Autodesk Inventor part; units mm, degrees
ref_plane "YZ Plane" through (0, 0, 0) normal (1, 0, 0) x (0, 1, 0)
ref_plane "XZ Plane" through (0, 0, 0) normal (0, 1, 0) x (-1, 0, 0)
ref_plane "XY Plane" through (0, 0, 0) normal (0, 0, 1) x (1, 0, 0)
sketch "草图1" plane through (0, 0, 0) normal (0, 1, 0) x (-1, 0, 0)
  line L0 (0, 0) -> (-8, 0)
  line L1 (-8, 0) -> (-8, -5)
  line L2 (-8, -5) -> (0, -5)
  line L3 (0, -5) -> (0, 0)
  line L4 (0, -5) -> (-5, -5)
  line L5 (-5, -5) -> (-5, -7.5)
  line L6 (-5, -7.5) -> (0, -7.5)
  line L7 (0, -7.5) -> (0, -5)
  line L8 (0, -7.5) -> (-5.75, -7.5)
  line L9 (-5.75, -7.5) -> (-5.75, -45)
  line L10 (-5.75, -45) -> (0, -45)
  line L11 (0, -45) -> (0, -7.5)
  line L12 (0, -45) -> (-5.25, -45)
  line L13 (-5.25, -45) -> (-5.25, -46.1)
  line L14 (-5.25, -46.1) -> (0, -46.1)
  line L15 (0, -46.1) -> (0, -45)
  line L16 (0, -46.1) -> (-5.75, -46.1)
  line L17 (-5.75, -46.1) -> (-5.75, -50)
  line L18 (-5.75, -50) -> (0, -50)
  line L19 (0, -50) -> (0, -46.1)
  dimension "d0" = 8
  dimension "d1" = 5
  dimension "d2" = 5
  dimension "d3" = 2.5
  dimension "d4" = 5.75
  dimension "d5" = 37.5
  dimension "d6" = 5.25
  dimension "d7" = 1.1
  dimension "d8" = 5.75
  dimension "d9" = 3.9
revolve "旋转1" add sketch "草图1" angle 360 about axis through (0, 0, -45) along (0, 0, 1)
fillet "圆角1" radius 1 2 edges at (-8, 0, 0) (-5.75, 0, -50)
properties part number "6-鞘轴" material "不锈钢"
Source: CAD feature listing. Evaluate the final solid. Frame: model axes, mm. A direction names the side the tool comes from. Give positions to 0.01 mm unless a question says otherwise; leave off trailing zeros. Order: outer loops, then holes, each group sorted by start corner. A loop starts at its lowest first (then second) coordinate and runs counter-clockwise, first axis right, second up. Notation, with made-up numbers: (7.5, -38) -> (65.5, -38) arc R12 cw to (65.5, -29) -> close; hole circle Ø2 at (84, 53). An arc over 180 degrees is marked (long way). Write item = value, one per line.
Q1. Pin query (flat end, axial travel): pin 1 (8 mm diameter, centred on y = -3, z = -19, fed in from +X); pin 2 (4 mm diameter, centred on y = 6, z = -11.5, fed in from -X); pin 3 (2 mm diameter, centred on x = 0, z = -45, fed in from +Y). Return the tip coordinate at first contact, or that it passes through.
Data:
pin_1 = 5.75
pin_2 = -4.13
pin_3 = 5.75
Q2. Cut plane A-A, the plane x = 0. Output: boundary loops of the cut face in (y, z), and give its area (3 significant figures).
Data:
outline = (-8, -5) -> (-5, -5) -> (-5, -7.5) -> (-5.75, -7.5) -> (-5.75, -45) -> (-5.25, -45) -> (-5.25, -46.1) -> (-5.75, -46.1) -> (-5.75, -49) arc R1 ccw to (-4.75, -50) -> (4.75, -50) arc R1 ccw to (5.75, -49) -> (5.75, -46.1) -> (5.25, -46.1) -> (5.25, -45) -> (5.75, -45) -> (5.75, -7.5) -> (5, -7.5) -> (5, -5) -> (8, -5) -> (8, -1) arc R1 ccw to (7, 0) -> (-7, 0) arc R1 ccw to (-8, -1) -> close
area = 592 mm^2
Q3. Set-up query: faces 1 (the face through (5, -1.6, -45.6)), 2 (the face through (-0.75, -5.7, -26.51)), 3 (the face through (-1.73, 7.81, -3.03)). Return all of +Z, -Z, +X, -X, +Y, -Y with unobstructed straight access to the full face (end or side cutting, diameter ignored); none if empty.
Data:
face_1 = none
face_2 = -Z
face_3 = +Z, -Z
Q4. Cut plane C-C, the plane z = -3. Output: boundary loops of the cut face in (x, y), and give its area (3 significant figures).
Data:
outline = circle Ø16 at (0, 0)
area = 201 mm^2
Q5. Material intervals for line 1 (Z direction, x = 1, y = -7); line 2 (X direction, y = -0.25, z = -6); line 3 (Z direction, x = -4.25, y = -3), sorted ascending. Write a range as from..to.
Data:
line_1 = -5..0
line_2 = -4.99..4.99
line_3 = -49.89..-7.5, -5..0
Q6. Pull-direction query (Z, two-part tool) for faces 4 (the face through (-1.08, 4.88, -6.27)), 5 (the face through (-0.75, -5.7, -47.57)), 6 (the face through (0, 0, 0)), 7 (the face through (0, 0, -50)); classes: released by +Z, released by -Z, zero draft, split by the parting line, or undercut.
Data:
face_4 = undercut
face_5 = zero draft
face_6 = released by +Z
face_7 = released by -Z
Q7. Cut plane D-D, the plane z = -40. Output: boundary loops of the cut face in (x, y), and give its area (3 significant figures).
Data:
outline = circle Ø11.5 at (0, 0)
area = 104 mm^2
